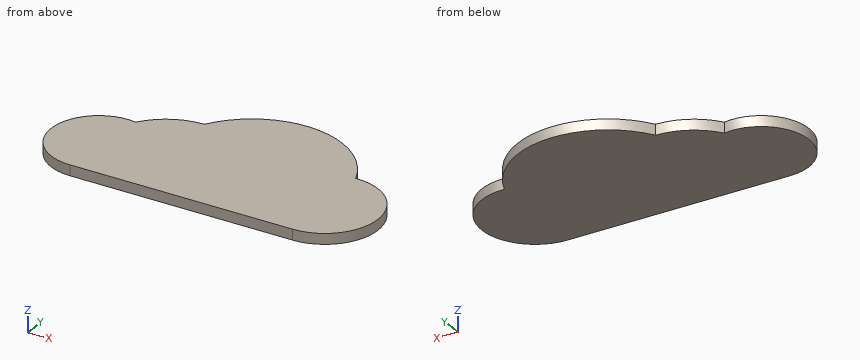
from build123d import *

# Parameters (mm, degrees)
PAD_DEPTH = 2.54


with BuildPart() as part:
    # Sketch → Pad (new body)
    with BuildSketch(Plane.XY):
        with BuildLine():
            ThreePointArc((30.679575, 60.787624), (17.315176, 50.522537), (28.702, 38.1))
            Line((28.702, 38.1), (82.042, 38.1))
            ThreePointArc((82.042, 38.1), (94.740642, 50.985703), (81.670634, 63.494569))
            ThreePointArc((81.670634, 63.494569), (63.596138, 77.364858), (43.151783, 67.309974))
            ThreePointArc((43.151783, 67.309974), (36.117636, 65.574837), (30.679575, 60.787624))
        make_face()
    extrude(amount=PAD_DEPTH)


solid = part.part
Geometry check sheet. Reference: the model listing, model coordinates, mm. Coordinates: 2 decimals unless noted, no trailing zeros. Loops run counter-clockwise (first coordinate to the right, second up) from the corner with the lowest first, then second, coordinate; pieces in that order, holes last. Notation, with made-up numbers: (-16, 11) - (25, 11) arc R10 ccw to (25, 19) - close; hole circle Ø1 at (45, 71). An arc over 180 degrees is marked (long way). Use one line per item in the form item = value. Start each with the question number.
Item 1: Section check A-A, the plane z = 0.5. Enter the section's corners in (x, y).
Item 2: Section check B-B, the plane y = 43.5. Enter the section's corners in (x, z), and give its area (3 significant figures).
Item 3: Section check C-C, the plane x = 45. Enter the section's corners in (y, z).
Item 4: Thickness scan on probe 1 along Y at (x, z) = (29, 1.4); probe 2 along X at (y, z) = (64, 2.2); probe 3 along Y at (x, z) = (83, 2.1). Record the ranges inside material, lowest first.
Computed:
q1.outline = (28.7, 38.1) - (82.04, 38.1) arc R12.7 ccw (long way) to (81.67, 63.49) arc R21.59 ccw to (43.15, 67.31) arc R15.24 ccw to (30.68, 60.79) arc R11.43 ccw (long way) to start
q2.outline = (18.99, 0) - (92.43, 0) - (92.43, 2.54) - (18.99, 2.54) - close
q2.area = 187 mm2
q3.outline = (38.1, 0) - (69.84, 0) - (69.84, 2.54) - (38.1, 2.54) - close
q4.probe_1 = 38.1 to 60.96
q4.probe_2 = 33.7 to 81.47
q4.probe_3 = 38.14 to 63.46
